from build123d import *

# Parameters (mm, degrees)
SKETCH_1_W      = 20
SKETCH_1_H      = 55
EXTRUDE_1_DEPTH = 0.5
EXTRUDE_2_DEPTH = 20


with BuildPart() as part:
    # 草图1 → 凸台-拉伸1 (new body)
    with BuildSketch(Plane.XY):
        Rectangle(SKETCH_1_W, SKETCH_1_H)
    extrude(amount=EXTRUDE_1_DEPTH)

    # 草图2 → 凸台-拉伸2 (add)
    with BuildSketch(Plane.ZY.offset(10)):
        with BuildLine():
            Line((2.156267732, 30.305392831), (39.659750235, 44.215417999))
            Line((39.659750235, 44.215417999), (39.833625549, 43.746624468))
            Line((39.833625549, 43.746624468), (2.330143047, 29.8365993))
            add(Edge.make_bspline(
                [(0.5, 27.5), (0.5, 27.655778728), (0.711024801, 29.04730174), (1.493571631, 29.52631533), (2.330143047, 29.8365993)],
                knots=[0, 0, 0, 0, 0.26712767, 1, 1, 1, 1], degree=3))
            Line((0.5, 27.5), (0, 27.5))
            add(Edge.make_bspline(
                [(0, 27.5), (0, 27.638670788), (0.031716688, 27.88649079), (0.142334357, 28.422460253), (0.331831028, 28.912835815), (0.685759589, 29.46438852), (1.285915439, 29.952226685), (1.865336089, 30.197486413), (2.156267732, 30.305392831)],
                knots=[0, 0, 0, 0, 0.125, 0.25, 0.375, 0.5, 0.75, 1, 1, 1, 1], degree=3))
        make_face()
    extrude(amount=-EXTRUDE_2_DEPTH)


solid = part.part
Source: CAD feature listing. Evaluate the final solid. Frame: model axes, mm. A direction names the side the tool comes from. Give positions to 0.01 mm unless a question says otherwise; leave off trailing zeros. Write each loop counter-clockwise with the first axis right and the second up, starting at its lowest first coordinate (ties: lowest second). Pieces come first, ordered by that corner, then holes. Notation, with made-up numbers: M -22.75,0.25 L -8.75,0.25 A20 cw -8.75,6.25 Z; hole C -32,-21 d5. An arc over 180 degrees is marked long. Return JSON: item names as keys, results as strings. Group by question number.
1) Material intervals for line 1 along Z through (x, y) = (2, 21); line 2 along Y through (x, z) = (-4.5, 7.5); line 3 along Y through (x, z) = (2.75, 24), sorted ascending. Write a range as [from, to].
2) Set-up query: faces 1 (the face through (0, 0, 0.5)), 2 (the face through (-0.14, 37.163, 20.645)). Return all of +Z, -Z, +X, -X, +Y, -Y with unobstructed straight access to the full face (end or side cutting, diameter ignored); none if empty.
3) Pin query (flat end, axial travel): P1, Ø8, axis at y = 0.5, z = 5.5, coming from the -X side; P2, Ø2, axis at x = -3.5, z = 19, coming from the -Y side; P3, Ø12, axis at x = -2, y = 10.5, coming from the -Z side; P4, Ø5, axis at x = 6, z = 17.5, coming from the +Y side. Return the tip coordinate at first contact, or that it passes through.
4) Cut plane A-A, the plane y = 15. Output: boundary loops of the cut face in (x, z).
5) Cut plane B-B, the plane z = 16.5. Output: boundary loops of the cut face in (x, y), plus the area to 3 significant figures.
Recorded:
{
 "1": {"line 1": "z = [0, 0.5]", "line 2": "y = [31.75, 32.29]", "line 3": "y = [37.87, 38.41]"},
 "2": {"face 1": "+Z, +X, -X, -Y", "face 2": "-Z, +X, -X, +Y"},
 "3": {"P1": "passes through", "P2": "stops at y = 35.65", "P3": "stops at z = 0", "P4": "stops at y = 36.92"},
 "4": {"outline": "M -10,0 L 10,0 L 10,0.5 L -10,0.5 Z"},
 "5": {"outline": "M -10,35.09 L 10,35.09 L 10,35.63 L -10,35.63 Z", "area": "10.7 mm²"}
}
